```python
from build123d import *

# Parameters (mm, degrees)
BOSS_EXTRUDE1_DEPTH = 40
SKETCH2_W           = 154.782746008
SKETCH2_H           = 50
CUT_EXTRUDE1_DEPTH  = 44.884825983
SKETCH2_2_W         = 154.782746008
SKETCH2_2_H         = 50
CUT_EXTRUDE2_DEPTH  = 27.115174017
SKETCH3_R           = 15
BOSS_EXTRUDE2_DEPTH = 3
SKETCH4_R           = 30
BOSS_EXTRUDE3_DEPTH = 10
SKETCH5_R           = 25
BOSS_EXTRUDE4_DEPTH = 3
FILLET1_R           = 100
FILLET2_R           = 100
FILLET3_R           = 10


with BuildPart() as part:
    # Sketch1 → Boss-Extrude1 (new body, symmetric)
    with BuildSketch(Plane.XY):
        with BuildLine():
            Line((-54.159677949, -43.884825983), (40.108572858, -43.884825983))
            Line((40.108572858, -43.884825983), (71.049767381, -38.429058573))
            ThreePointArc((71.049767381, -38.429058573), (95.840322051, -8.884825983), (71.049767381, 20.659406608))
            Line((71.049767381, 20.659406608), (40.108572858, 26.115174017))
            Line((40.108572858, 26.115174017), (-54.159677949, 26.115174017))
            Line((-54.159677949, 26.115174017), (-54.159677949, -43.884825983))
        make_face()
    extrude(amount=BOSS_EXTRUDE1_DEPTH, both=True)

    # Sketch2 → Cut-Extrude1 (cut, through all)
    with BuildSketch(Plane(origin=(0, 0, 0), x_dir=(1, 0, 0), z_dir=(0, 1, 0))):
        with Locations((43.231695055, 0)):
            Rectangle(SKETCH2_W, SKETCH2_H)
    extrude(amount=-CUT_EXTRUDE1_DEPTH, mode=Mode.SUBTRACT)

    # Sketch2<2> → Cut-Extrude2 (cut, through all)
    with BuildSketch(Plane(origin=(0, 0, 0), x_dir=(1, 0, 0), z_dir=(0, 1, 0))):
        with Locations((43.231695055, 0)):
            Rectangle(SKETCH2_2_W, SKETCH2_2_H)
    extrude(amount=CUT_EXTRUDE2_DEPTH, mode=Mode.SUBTRACT)

    # Sketch3 → Boss-Extrude2 (add)
    with BuildSketch(Plane.XY.offset(-25)):
        with Locations((65.840322051, -8.884825983)):
            Circle(SKETCH3_R)
    boss_extrude2 = extrude(amount=BOSS_EXTRUDE2_DEPTH)

    # Mirror1: Boss-Extrude2 across plane
    add(boss_extrude2.mirror(Plane.XY))

    # Sketch4 → Boss-Extrude3 (add)
    with BuildSketch(Plane.ZY.offset(54.159677949)):
        with Locations((0, -8.884825983)):
            Circle(SKETCH4_R)
    extrude(amount=BOSS_EXTRUDE3_DEPTH)

    # Sketch5 → Boss-Extrude4 (add)
    with BuildSketch(Plane.ZY.offset(64.159677949)):
        with Locations((0, -8.884825983)):
            Circle(SKETCH5_R)
    extrude(amount=BOSS_EXTRUDE4_DEPTH)

    # Fillet1
    fillet1_edges = [part.edges().sort_by_distance(p)[0] for p in [
        (40.108572858, 26.115174017, 32.5),
        (40.108572858, 26.115174017, -32.5),
    ]]
    fillet(fillet1_edges, radius=FILLET1_R)

    # Fillet2
    fillet2_edges = [part.edges().sort_by_distance(p)[0] for p in [
        (40.108572858, -43.884825983, 32.5),
        (40.108572858, -43.884825983, -32.5),
    ]]
    fillet(fillet2_edges, radius=FILLET2_R)

    # Fillet3
    fillet3_edges = [part.edges().sort_by_distance(p)[0] for p in [
        (-34.159677949, -8.884825983, -25),
        (-34.159677949, -8.884825983, 25),
    ]]
    fillet(fillet3_edges, radius=FILLET3_R)


solid = part.part
```
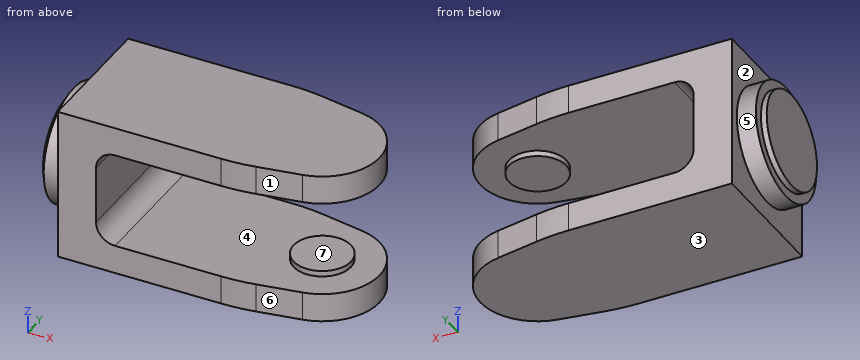
CAD build for the part. Positions are in the model's coordinates, mm. Face numbers are marked on the shaded views. A direction names the side the tool comes from. Give positions to 0.01 mm unless a question says otherwise; leave off trailing zeros. Loops run counter-clockwise (first coordinate to the right, second up) from the corner with the lowest first, then second, coordinate; pieces in that order, holes last. Notation, with made-up numbers: (55.25, 5) -> (71.25, 5) arc R24 ccw to (71.25, 17) -> close; hole circle Ø10 at (8.25, -22.75). An arc over 180 degrees is marked (long way). Use a Markdown table: item, result.
1. Slice it at B-B (z = 0). List the corners of the cut face in (x, y), plus the area to 3 significant figures.
Check result:
| item | result |
|---|---|
| outline | (-67.16, -33.88) -> (-64.16, -33.88) -> (-64.16, -38.88) -> (-54.16, -38.88) -> (-54.16, -43.88) -> (-34.16, -43.88) -> (-34.16, 26.12) -> (-54.16, 26.12) -> (-54.16, 21.12) -> (-64.16, 21.12) -> (-64.16, 16.12) -> (-67.16, 16.12) -> close |
| area | 2,150 mm^2 |
2. Slice it at A-A (x = -7.5). List the corners of the cut face in (y, z).
Check result:
| item | result |
|---|---|
| outline | (-43.88, -40) -> (26.12, -40) -> (26.12, -25) -> (-43.88, -25) -> close; (-43.88, 25) -> (26.12, 25) -> (26.12, 40) -> (-43.88, 40) -> close |
3. Flat gauge pins, fed straight in: pin 1 (6 mm diameter, centred on y = 12, z = 27.5, fed in from -X); pin 2 (12 mm diameter, centred on x = 45.5, z = -29.5, fed in from +Y); pin 3 (24 mm diameter, centred on y = -3, z = -5, fed in from +X). Where does each tip first touch, or does it go through?
Check result:
| item | result |
|---|---|
| pin 1 | stops at x = -54.16 |
| pin 2 | stops at y = 25.78 |
| pin 3 | stops at x = -33.96 |
4. Mould opens along X. For the marked faces 1, 2, 3 and 4 say: pulls with the +X half, pulls with the -X half, needs draft (parallel to the pull), parting line crosses it, or undercut.
Check result:
| item | result |
|---|---|
| face 1 | pulls with the +X half |
| face 2 | pulls with the -X half |
| face 3 | needs draft |
| face 4 | undercut |
5. Wall check: L1, parallel to Z at x = 57.5, y = -20; L2, parallel to Z at x = 49, y = -17; L3, parallel to X at y = 9, z = 12.5. Give the ranges that are in metal, low to high. Write a range as [from, to].
Check result:
| item | result |
|---|---|
| L1 | z = [-40, -22], [22, 40] |
| L2 | z = [-40, -25], [25, 40] |
| L3 | x = [-67.16, -34.16] |
6. Slice it at D-D (x = 65). List the corners of the cut face in (y, z), plus the area to 3 significant figures.
Check result:
| item | result |
|---|---|
| outline | (-39.5, -40) -> (21.73, -40) -> (21.73, -25) -> (6.09, -25) -> (6.09, -22) -> (-23.86, -22) -> (-23.86, -25) -> (-39.5, -25) -> close; (-39.5, 25) -> (-23.86, 25) -> (-23.86, 22) -> (6.09, 22) -> (6.09, 25) -> (21.73, 25) -> (21.73, 40) -> (-39.5, 40) -> close |
| area | 2,020 mm^2 |
7. Slice it at C-C (y = -11). List the corners of the cut face in (x, z).
Check result:
| item | result |
|---|---|
| outline | (-67.16, -24.91) -> (-64.16, -24.91) -> (-64.16, -29.93) -> (-54.16, -29.93) -> (-54.16, -40) -> (95.77, -40) -> (95.77, -25) -> (80.69, -25) -> (80.69, -22) -> (50.99, -22) -> (50.99, -25) -> (-24.16, -25) arc R10 cw to (-34.16, -15) -> (-34.16, 15) arc R10 cw to (-24.16, 25) -> (50.99, 25) -> (50.99, 22) -> (80.69, 22) -> (80.69, 25) -> (95.77, 25) -> (95.77, 40) -> (-54.16, 40) -> (-54.16, 29.93) -> (-64.16, 29.93) -> (-64.16, 24.91) -> (-67.16, 24.91) -> close |
8. Which spindle directions (+Z, -Z, +X, -X, +Y, -Y) get a long thin tool onto all of the face, cutting with end or side? Do the marked faces 5, 6 and 7. Say none if no direction does.
Check result:
| item | result |
|---|---|
| face 5 | -X |
| face 6 | +Z, -Z, +X, -Y |
| face 7 | +X, +Y, -Y |
